Model file for the job. Use its own axes, mm. A direction names the side the tool comes from. Give positions to 0.01 mm unless a question says otherwise; leave off trailing zeros. Loops run counter-clockwise (first coordinate to the right, second up) from the corner with the lowest first, then second, coordinate; pieces in that order, holes last. Notation, with made-up numbers: (69, 15) - (102, 15) arc R20 cw to (102, 19) - close; hole circle Ø7 at (73.5, 10). An arc over 180 degrees is marked (long way). Use a Markdown table: item, result.
Autodesk Inventor part; units mm, degrees
ref_plane "YZ Plane" through (0, 0, 0) normal (1, 0, 0) x (0, 1, 0)
ref_plane "XZ Plane" through (0, 0, 0) normal (0, 1, 0) x (-1, 0, 0)
ref_plane "XY Plane" through (0, 0, 0) normal (0, 0, 1) x (1, 0, 0)
sketch "Esboço1" plane through (0, 0, 0) normal (0, 1, 0) x (-1, 0, 0)
  line L0 (9.4987, -2.4377) -> (-20.5013, -2.4377)
  line L1 (-20.5013, -2.4377) -> (-20.5013, -42.4377)
  line L2 (-20.5013, -42.4377) -> (9.4987, -42.4377)
  line L3 (9.4987, -42.4377) -> (9.4987, -2.4377)
  point P0 (0, 0)
  dimension "d0" = 30
  dimension "d1" = 40
extrude "Extrusão1" add sketch "Esboço1" along normal blind 18
sketch "Esboço2" plane through (20.5013, 0, -42.4377) normal (0, 0, -1) x (-1, 0, 0)
  line L0 (28, 2) -> (2, 2)
  line L1 (2, 2) -> (2, 16)
  line L2 (2, 16) -> (28, 16)
  line L3 (28, 16) -> (28, 2)
  line L4 (0, 0) -> (30, 0)
  line L5 (0, 18) -> (30, 18)
  line L6 (0, 0) -> (0, 18)
  line L7 (30, 0) -> (30, 18)
  point P0 (20.5013, 0)
  dimension "d4" = 2
  dimension "d5" = 2
  dimension "d6" = 2
  dimension "d7" = 2
extrude "Extrusão2" cut sketch "Esboço2" against normal blind 38 contours L0 L1 L2 L3
chamfer "Chanfro1" distance 2 angle 45 7 edges at (-9.4987, 18, -22.4377) (-9.4987, 0, -22.4377) (5.5013, 18, -2.4377) (-9.4987, 9, -2.4377) (20.5013, 18, -22.4377) (20.5013, 9, -2.4377) (20.5013, 0, -22.4377)
chamfer "Chanfro2" distance 2 angle 45 1 edges at (5.5013, 0, -2.4377)
sketch "Esboço3" plane through (0, 0, 0) normal (0, -1, 0) x (1, 0, 0)
  line L0 (-3.4987, -6.1642) -> (14.5013, -6.1642)
  line L1 (14.5013, -6.1642) -> (14.5013, -24.1642)
  line L2 (14.5013, -24.1642) -> (-3.4987, -24.1642)
  line L3 (-3.4987, -24.1642) -> (-3.4987, -6.1642)
  line L4 (-7.4987, -42.4377) -> (-7.4987, -4.4377)
  point P0 (0, 0)
  dimension "d16" = 18
  dimension "d17" = 18
  dimension "d18" = 4
extrude "Extrusão3" cut sketch "Esboço3" against normal blind 5
sketch "Esboço4" plane through (-9.4987, 2, -42.4377) normal (-1, 0, 0) x (0, 0, 1)
  line L0 (0, 14) -> (38, 14)
  line L1 (7.7786, 13) -> (0, 13)
  line L2 (7.7786, 1) -> (0, 1)
  line L3 (0, 0) -> (0, 14)
  ellipse E0 centre (13.7786, 7) end of major axis (13.7786, 10) minor radius 3.3 (13.0203, 4.0803) -> (13.0203, 9.9197) ccw
  arc A0 (7.7786, 1) -> (13.0203, 4.0803) centre (7.7786, 7) ccw
  arc A1 (13.0203, 9.9197) -> (7.7786, 13) centre (7.7786, 7) ccw
  circle A2 centre (7.7786, 7) radius 2
  point P0 (42.4377, -2)
  dimension "d23" = 3.3
  dimension "d24" = 3
  dimension "d22" = 7
  dimension "d25" = 4
extrude "Extrusão4" cut sketch "Esboço4" against normal blind 5
sketch "Esboço5" plane through (-9.4987, 9, -34.6591) normal (-1, 0, 0) x (0, 0, 1)
  circle A0 centre (0, 0) radius 2
  circle A1 centre (0, 0) radius 2
  point P0 (34.6591, -9)
extrude "Extrusão5" cut sketch "Esboço5" against normal blind 69
sketch "Esboço6" plane through (-7.4987, 16, -2.4377) normal (0, 0, 1) x (1, 0, 0)
  line L0 (0, -4) -> (0, -10) construction
  line L1 (0, -7) -> (26, -7) construction
  line L2 (26, -9) -> (26, -5) construction
  line L3 (22, -14) -> (4, -14) construction
  line L4 (13, -14) -> (13, 0) construction
  line L5 (26, 0) -> (0, 0) construction
  circle A0 centre (13, -7) radius 2
  point P0 (7.4987, -16)
  point P1 (0, -9.9197)
  point P2 (0, -4.0803)
  dimension "d30" = 4
extrude "Extrusão6" cut sketch "Esboço6" against normal blind 10
properties part number "Pernotta"
(1) Pin check, flat tips, straight feed: P1, Ø0.6, axis at x = -8, z = -38, coming from the -Y side; P2, Ø1, axis at x = 13.5, y = 9.5, coming from the -Z side; P3, Ø4.5, axis at y = 9, z = -34.66, coming from the -X side; P4, Ø3, axis at x = 5.5, y = 9, coming from the +Z side. Stop position of each tip, or through.
Computed:
| item | result |
|---|---|
| P1 | y = 0.2 |
| P2 | z = -4.44 |
| P3 | x = 18.5 |
| P4 | through |
(2) 3-axis set-ups, long thin cutter, end or side, ignore diameter. For faces 4 (the flat face through (14.501, 1, -15)), 5 (the flat face through (6, 16, -24)), 6 (the flat face through (-9.499, 9, -19)), 7 (the flat face through (-9, 15, -38)), 8 (the flat face through (-8.48, 8.6, -3.42)): which of +Z, -Z, +X, -X, +Y, -Y reach the whole face in a straight line?
Computed:
| item | result |
|---|---|
| face 4 | -Y |
| face 5 | -Z |
| face 6 | +Z, -Z, -X, +Y, -Y |
| face 7 | -Z, -X |
| face 8 | +Z, -X, +Y, -Y |
(3) Slice it at B-B, the plane x = -4.5. Write the cut outline in (y, z), plus the area to 3 significant figures.
Computed:
| item | result |
|---|---|
| outline | (0, -42.44) - (2, -42.44) - (2, -4.44) - (16, -4.44) - (16, -42.44) - (18, -42.44) - (18, -4.44) - (16, -2.44) - (2, -2.44) - (0, -4.44) - close |
| area | 184 mm² |
(4) Mould opens along Z. For faces 1 (the flat face through (5.68, 17.01, -3.45)), 2 (the cylindrical face through (-8.513, 3.805, -31.658)), 3 (the flat face through (5, 1, -6.164)) say: pulls with the +Z half, pulls with the -Z half, needs draft (parallel to the pull), parting line crosses it, or undercut.
Computed:
| item | result |
|---|---|
| face 1 | pulls with the +Z half |
| face 2 | pulls with the -Z half |
| face 3 | undercut |
(5) Slice it at D-D, the plane y = 9. Count the separate pieces of the cut face and the enclosed holes in it, plus the area to 3 significant figures.
Computed:
| item | result |
|---|---|
| separate pieces | 3 |
| enclosed holes | 0 |
| area | 158 mm² |
(6) Slice it at A-A, the plane x = 2.5. Write the cut outline in (y, z), plus the area to 3 significant figures.
Computed:
| item | result |
|---|---|
| outline | (0, -42.44) - (2, -42.44) - (2, -24.16) - (0, -24.16) - close; (0, -6.16) - (2, -6.16) - (2, -4.44) - (16, -4.44) - (16, -42.44) - (18, -42.44) - (18, -4.44) - (16, -2.44) - (2, -2.44) - (0, -4.44) - close |
| area | 148 mm² |
(7) Drill centre lines: probe 1 along X at (y, z) = (2.5, -20); probe 2 along Y at (x, z) = (6.5, -38.5); probe 3 along Z at (x, y) = (10.5, 3). Where is each one in solid material? Low to high. Write a range as [from, to].
Computed:
| item | result |
|---|---|
| probe 1 | [-9.5, -7.5], [18.5, 20.5] |
| probe 2 | [0, 2], [16, 18] |
| probe 3 | [-4.44, -2.44] |
(8) Slice it at C-C, the plane y = 12.75. Write the cut outline in (x, z), plus the area to 3 significant figures.
Computed:
| item | result |
|---|---|
| outline | (-9.5, -29.98) - (-7.5, -29.98) - (-7.5, -4.44) - (18.5, -4.44) - (18.5, -42.44) - (20.5, -42.44) - (20.5, -4.44) - (18.5, -2.44) - (-7.5, -2.44) - (-9.5, -4.44) - close |
| area | 183 mm² |
